Input: dimensioned drawing with shaded views. Units: mm. Origin: part minimum x, y, z. A direction names the side the tool comes from. Round coordinates to 2 decimals unless told otherwise and drop trailing zeros. Order: outer loops, then holes, each group sorted by start corner. A loop starts at its lowest first (then second) coordinate and runs counter-clockwise, first axis right, second up. Notation, with made-up numbers: M -22.5,25.25 L 28.5,25.25 A11 cw 28.5,42.25 Z; hole C 80,-16 d8. An arc over 180 degrees is marked long. Put each result on its own line as item: value. Start each with the question number.
1) Section C-C, the plane y = 2. Return loops of the section in (x, z), then the cut area to 3 significant figures.
2) Section D-D, the plane z = 7.25. Return loops of the section in (x, y), then the cut area to 3 significant figures.
3) Section B-B, the plane z = 4. Return loops of the section in (x, y), then the cut area to 3 significant figures.
4) Material intervals for probe 1 along X at (y, z) = (0.25, 4); probe 2 along X at (y, z) = (3.8, 5); probe 3 along X at (y, z) = (2.8, 4), sorted ascending. Write a range as [from, to].
5) First-contact query: P1, Ø1, axis at x = 5.5, y = 3, coming from the +Z side. Flat tip, straight axial feed; report the tip coordinate or a pass-through.
6) Section A-A, the plane x = 4. Return loops of the section in (y, z), then the cut area to 3 significant figures.
7) Access query for the marked faces 4 and 5. Directions: +Z, -Z, +X, -X, +Y, -Y. A direction counts if a zero-diameter tool reaches every point of the face in a straight line with its end or side. Return the directions, or none.
8) Draft query along Z for the marked faces 1, 2 and 3. Return one class per face: pulls with the +Z half, pulls with the -Z half, needs draft (parallel to the pull), parting line crosses it, or undercut.
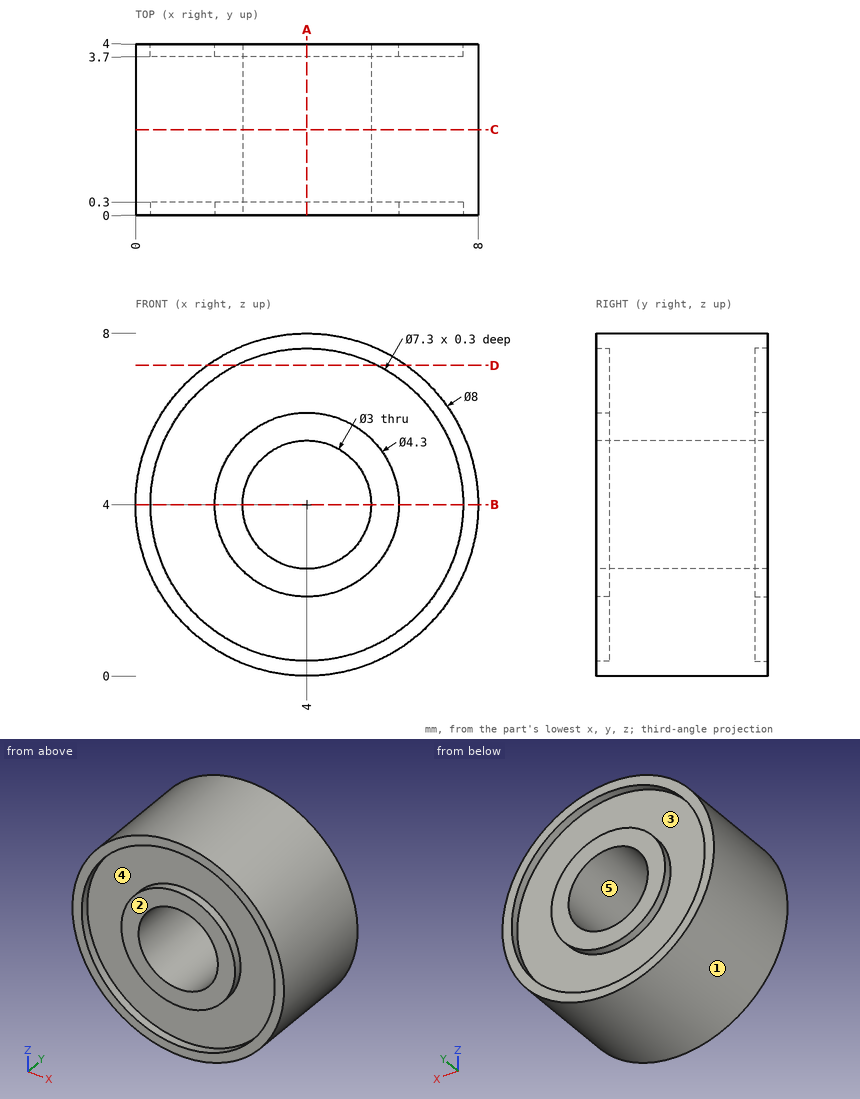
Result sheet:
1. outline: C 4,4 d8; hole C 4,4 d3
1. area: 43.2 mm2
2. outline: M 1.67,0 L 2.34,0 L 2.34,0.3 L 5.66,0.3 L 5.66,0 L 6.33,0 L 6.33,4 L 5.66,4 L 5.66,3.7 L 2.34,3.7 L 2.34,4 L 1.67,4 Z
2. area: 16.7 mm2
3. outline: M 0,0 L 0.35,0 L 0.35,0.3 L 1.85,0.3 L 1.85,0 L 2.5,0 L 2.5,4 L 1.85,4 L 1.85,3.7 L 0.35,3.7 L 0.35,4 L 0,4 Z; M 5.5,0 L 6.15,0 L 6.15,0.3 L 7.65,0.3 L 7.65,0 L 8,0 L 8,4 L 7.65,4 L 7.65,3.7 L 6.15,3.7 L 6.15,4 L 5.5,4 Z
3. area: 18.2 mm2
4. probe 1: x = [0, 0.35], [1.85, 2.5], [5.5, 6.15], [7.65, 8]
4. probe 2: x = [0.13, 0.49], [2.1, 2.88], [5.12, 5.9], [7.51, 7.87]
4. probe 3: x = [0, 2.5], [5.5, 8]
5. P1: stops at z = 7.87
6. outline: M 0,0 L 4,0 L 4,0.35 L 3.7,0.35 L 3.7,1.85 L 4,1.85 L 4,2.5 L 0,2.5 L 0,1.85 L 0.3,1.85 L 0.3,0.35 L 0,0.35 Z; M 0,5.5 L 4,5.5 L 4,6.15 L 3.7,6.15 L 3.7,7.65 L 4,7.65 L 4,8 L 0,8 L 0,7.65 L 0.3,7.65 L 0.3,6.15 L 0,6.15 Z
6. area: 18.2 mm2
7. face 4: -Y
7. face 5: +Y, -Y
8. face 1: parting line crosses it
8. face 2: needs draft
8. face 3: undercut
